Autodesk Inventor part; units mm, degrees
ref_plane "YZ Plane" through (0, 0, 0) normal (1, 0, 0) x (0, 1, 0)
ref_plane "XZ Plane" through (0, 0, 0) normal (0, 1, 0) x (-1, 0, 0)
ref_plane "XY Plane" through (0, 0, 0) normal (0, 0, 1) x (1, 0, 0)
sketch "Эскиз1" plane through (0, 0, 0) normal (0, 0, 1) x (1, 0, 0)
  line L0 (63.5, -82.5) -> (-63.5, -82.5)
  line L1 (-63.5, -82.5) -> (-63.5, 82.5)
  line L2 (63.5, 82.5) -> (63.5, -82.5)
  line L3 (-63.5, 82.5) -> (63.5, 82.5)
  point P0 (0, 0)
extrude "Выдавливание1" add sketch "Эскиз1" along normal blind 5
sketch "Эскиз2" plane through (0, 0, 0) normal (0, 0, 1) x (1, 0, 0)
  line L0 (-63.5, -82.5) -> (-63.5, 82.5)
  line L1 (-63.5, 82.5) -> (63.5, 82.5)
  line L2 (63.5, 82.5) -> (63.5, -82.5)
  line L3 (63.5, -82.5) -> (-63.5, -82.5)
  line L4 (-61.7, 80.7) -> (-61.7, -80.7)
  line L5 (-61.7, -80.7) -> (61.7, -80.7)
  line L6 (61.7, -80.7) -> (61.7, 80.7)
  line L7 (61.7, 80.7) -> (-61.7, 80.7)
  point P0 (0, 0)
  dimension "d2" = 1.8
extrude "Выдавливание2" add sketch "Эскиз2" against normal blind 2
properties part number "Крышка контейнера"
Here's how the part is built. I have some questions about the finished solid (model axes, mm). A direction names the side the tool comes from. Coordinates: 2 decimals unless noted, no trailing zeros. Order: outer loops, then holes, each group sorted by start corner. A loop starts at its lowest first (then second) coordinate and runs counter-clockwise, first axis right, second up. Notation, with made-up numbers: M 67,-9.75 L 118,-9.75 A14 cw 118,2.25 Z; hole C 73,28.5 d10. An arc over 180 degrees is marked long. Answer as CSV lines item,"result".
Item 1: Imagine slicing it at B-B on y = -36. Write out the boundary of the cut face in (x, z).
Results found:
outline,"M -63.5,-2 L -61.7,-2 L -61.7,0 L 61.7,0 L 61.7,-2 L 63.5,-2 L 63.5,5 L -63.5,5 Z"
Item 2: On a 3-axis mill with a long thin cutter (end or side, diameter ignored), from which of +Z, -Z, +X, -X, +Y, -Y can I reach the whole of each face in a straight line? I mean faces 1 (the face through (-1, 1, 5)), 2 (the face through (-1, 1, 0)). Say none if no direction works.
Results found:
face 1,"+Z, +X, -X, +Y, -Y"
face 2,"-Z"
Item 3: Imagine slicing it at A-A on x = -10. Write out the boundary of the cut face in (y, z).
Results found:
outline,"M -82.5,-2 L -80.7,-2 L -80.7,0 L 80.7,0 L 80.7,-2 L 82.5,-2 L 82.5,5 L -82.5,5 Z"
Item 4: If I drill on line 1 (X direction, y = -56, z = -0.75); line 2 (Z direction, x = 43.5, y = -41); line 3 (Y direction, x = -42, z = -0.75), over which ranges is the centre line in solid material (lowest first)?
Results found:
line 1,"-63.5 to -61.7, 61.7 to 63.5"
line 2,"0 to 5"
line 3,"-82.5 to -80.7, 80.7 to 82.5"
Item 5: For pin 1 (12 mm diameter, centred on x = -17, y = -50.5, fed in from -Z), with a flat end and sliding along its axis, tell me the tip position at first contact or that it passes through.
Results found:
pin 1,"z = 0"
